Input: part model. Units: mm. Frame: model coordinates. A direction names the side the tool comes from. Give positions to 0.01 mm unless a question says otherwise; leave off trailing zeros. Loops run counter-clockwise (first coordinate to the right, second up) from the corner with the lowest first, then second, coordinate; pieces in that order, holes last. Notation, with made-up numbers: (36.25, 25) -> (66.25, 25) arc R24 cw to (66.25, 62) -> close; hole circle Ø9 at (23, 57.5). An arc over 180 degrees is marked (long way). Answer as a JSON object with one key per item and string values.
```python
from build123d import *

# Parameters (mm, degrees)
SKETCH_1_W               = 265
SKETCH_1_H               = 165
EXTRUDE_1_DEPTH          = 64
EXTRUDE_2_DEPTH          = 8
CUT_EXTRUDE_1_DEPTH      = 185.820182881
CUT_EXTRUDE_1_DEPTH_BACK = 185.820182881
SKETCH_3_W               = 3
SKETCH_3_H               = 4
SKETCH_4_W               = 141
SKETCH_4_H               = 44
CUT_EXTRUDE_2_DEPTH      = 120


with BuildPart() as part:
    # 草图1 → 凸台-拉伸1 (new body)
    with BuildSketch(Plane(origin=(0, 0, 0), x_dir=(1, 0, 0), z_dir=(0, 1, 0))):
        Rectangle(SKETCH_1_W, SKETCH_1_H)
    extrude(amount=EXTRUDE_1_DEPTH)

    # 草图2 → 凸台-拉伸2 (add)
    with BuildSketch(Plane.XY.offset(82.5)):
        with BuildLine():
            Line((-132.5, 64), (-152.5, 64))
            Line((-152.5, 64), (-152.5, 35))
            Line((-152.5, 35), (-144.5, 35))
            ThreePointArc((-144.5, 35), (-141.5, 32), (-144.5, 29))
            Line((-144.5, 29), (-152.5, 29))
            Line((-152.5, 29), (-152.5, 0))
            Line((-152.5, 0), (-132.5, 0))
            Line((-132.5, 0), (-132.5, 64))
        make_face()
        with BuildLine():
            Line((152.5, 64), (132.5, 64))
            Line((132.5, 64), (132.5, 0))
            Line((132.5, 0), (152.5, 0))
            Line((152.5, 0), (152.5, 29))
            Line((152.5, 29), (144.5, 29))
            ThreePointArc((144.5, 29), (141.5, 32), (144.5, 35))
            Line((144.5, 35), (152.5, 35))
            Line((152.5, 35), (152.5, 64))
        make_face()
    extrude(amount=-EXTRUDE_2_DEPTH)

    # 草图3 → 切除-拉伸1 (cut, two sides: drawn at the far end of the back side and taken through both)
    with BuildSketch(Plane(origin=(0, 0, 0), x_dir=(0, 0, -1), z_dir=(1, 0, 0)).offset(-CUT_EXTRUDE_1_DEPTH_BACK)):
        with Locations((-70, 62)):
            Rectangle(SKETCH_3_W, SKETCH_3_H)
        with Locations((-63.833333333, 62)):
            Rectangle(SKETCH_3_W, SKETCH_3_H)
        with Locations((-57.666666667, 62)):
            Rectangle(SKETCH_3_W, SKETCH_3_H)
        with Locations((-51.5, 62)):
            Rectangle(SKETCH_3_W, SKETCH_3_H)
        with Locations((-45.333333333, 62)):
            Rectangle(SKETCH_3_W, SKETCH_3_H)
        with Locations((-39.166666667, 62)):
            Rectangle(SKETCH_3_W, SKETCH_3_H)
        with Locations((-33, 62)):
            Rectangle(SKETCH_3_W, SKETCH_3_H)
        with Locations((-26.833333333, 62)):
            Rectangle(SKETCH_3_W, SKETCH_3_H)
        with Locations((-20.666666667, 62)):
            Rectangle(SKETCH_3_W, SKETCH_3_H)
        with Locations((-14.5, 62)):
            Rectangle(SKETCH_3_W, SKETCH_3_H)
        with Locations((-8.333333333, 62)):
            Rectangle(SKETCH_3_W, SKETCH_3_H)
        with Locations((-2.166666667, 62)):
            Rectangle(SKETCH_3_W, SKETCH_3_H)
        with Locations((4, 62)):
            Rectangle(SKETCH_3_W, SKETCH_3_H)
        with Locations((10.166666667, 62)):
            Rectangle(SKETCH_3_W, SKETCH_3_H)
        with Locations((16.333333333, 62)):
            Rectangle(SKETCH_3_W, SKETCH_3_H)
        with Locations((22.5, 62)):
            Rectangle(SKETCH_3_W, SKETCH_3_H)
        with Locations((28.666666667, 62)):
            Rectangle(SKETCH_3_W, SKETCH_3_H)
        with Locations((34.833333333, 62)):
            Rectangle(SKETCH_3_W, SKETCH_3_H)
        with Locations((41, 62)):
            Rectangle(SKETCH_3_W, SKETCH_3_H)
        with Locations((47.166666667, 62)):
            Rectangle(SKETCH_3_W, SKETCH_3_H)
        with Locations((53.333333333, 62)):
            Rectangle(SKETCH_3_W, SKETCH_3_H)
        with Locations((59.5, 62)):
            Rectangle(SKETCH_3_W, SKETCH_3_H)
        with Locations((65.666666667, 62)):
            Rectangle(SKETCH_3_W, SKETCH_3_H)
        with Locations((71.833333333, 62)):
            Rectangle(SKETCH_3_W, SKETCH_3_H)
        with Locations((78, 62)):
            Rectangle(SKETCH_3_W, SKETCH_3_H)
    extrude(amount=CUT_EXTRUDE_1_DEPTH + CUT_EXTRUDE_1_DEPTH_BACK, mode=Mode.SUBTRACT)

    # 草图4 → 切除-拉伸2 (cut, symmetric)
    with BuildSketch(Plane(origin=(0, 0, 0), x_dir=(0, 0, -1), z_dir=(1, 0, 0))):
        with Locations((4, 30)):
            Rectangle(SKETCH_4_W, SKETCH_4_H)
    extrude(amount=CUT_EXTRUDE_2_DEPTH, both=True, mode=Mode.SUBTRACT)


solid = part.part
```
Q1. Section A-A, the plane y = 21. Return the cut outline in (x, z), then the cut area to 3 significant figures.
Evaluation:
{"outline": "(-152.5, 74.5) -> (-132.5, 74.5) -> (-132.5, -82.5) -> (132.5, -82.5) -> (132.5, 74.5) -> (152.5, 74.5) -> (152.5, 82.5) -> (-152.5, 82.5) -> close; hole (-120, -74.5) -> (120, -74.5) -> (120, 66.5) -> (-120, 66.5) -> close", "area": "10,200 mm2"}
Q2. Ray query, line 1 along X through (y, z) = (27, -31.5); line 2 along Y through (x, z) = (-54.5, -5); line 3 along Y through (x, z) = (-50.5, 25). Return the intervals inside material, ascending.
Evaluation:
{"line 1": "x = -132.5 to -120, 120 to 132.5", "line 2": "y = 0 to 8, 52 to 60", "line 3": "y = 0 to 8, 52 to 64"}
Q3. Access query for faces 1 (the flat face through (132.5, 32, -3)), 2 (the flat face through (-140, 32, 74.5)), 3 (the flat face through (-148, 29, 79)), 4 (the flat face through (2, 8, -3)). Directions: +Z, -Z, +X, -X, +Y, -Y. A direction counts if a zero-diameter tool reaches every point of the face in a straight line with its end or side. Return the directions, or none.
Evaluation:
{"face 1": "-Z, +X, +Y, -Y", "face 2": "-Z, -X, +Y, -Y", "face 3": "+Z, -Z, -X", "face 4": "none"}
Q4. Pin query (flat end, axial travel): pin 1 (5 mm diameter, centred on y = 34, z = -56, fed in from +X); pin 2 (0.9 mm diameter, centred on x = -27.5, z = 57.5, fed in from +Y). Return the tip coordinate at first contact, or that it passes through.
Evaluation:
{"pin 1": "stops at x = 132.5", "pin 2": "stops at y = 60"}
Q5. Draft query along Z for faces 5 (the flat face through (-2, 32, 82.5)), 6 (the flat face through (2, 52, -3)), 7 (the flat face through (-2, 0, 1)), 8 (the flat face through (140, 32, 74.5)). Return one class per face: +Z half, -Z half, draft (parallel to the pull), parting line (faces both ways), or undercut.
Evaluation:
{"face 5": "+Z half", "face 6": "undercut", "face 7": "draft", "face 8": "-Z half"}
Q6. Section B-B, the plane y = 56.5. Return the cut outline in (x, z).
Evaluation:
{"outline": "(-152.5, 74.5) -> (-132.5, 74.5) -> (-132.5, -82.5) -> (132.5, -82.5) -> (132.5, 74.5) -> (152.5, 74.5) -> (152.5, 82.5) -> (-152.5, 82.5) -> close"}
